Geometry check sheet. Reference: the model listing, model coordinates, mm. Face numbers are marked on the shaded views. Coordinates: 2 decimals unless noted, no trailing zeros. Write each loop counter-clockwise with the first axis right and the second up, starting at its lowest first coordinate (ties: lowest second). Pieces come first, ordered by that corner, then holes. Notation, with made-up numbers: (24, 2) -> (77, 2) arc R27 cw to (77, 41) -> close; hole circle Ø4 at (87, 89). An arc over 180 degrees is marked (long way). Answer as CSV lines item,"result".
```python
from build123d import *

# Parameters (mm, degrees)
EXTRUDE_1_DEPTH     = 3.6
SKETCH_2_W          = 40
SKETCH_2_H          = 20
CUT_EXTRUDE_1_DEPTH = 10


with BuildPart() as part:
    # 草图1 → 凸台-拉伸1 (new body)
    with BuildSketch(Plane.XY):
        Polygon((-95, 75.172935312), (-74.85, 75.172935312), (-74.85, 78.772935312), (-27.35, 78.772935312), (-27.35, 75.172935312), (20.15, 75.172935312), (20.15, 78.772935312), (67.65, 78.772935312), (67.65, 75.172935312), (87.799257887, 75), (87.799257887, 56.25), (91.399257887, 56.25), (91.399257887, 18.75), (87.799257887, 18.75), (87.799257887, -18.75), (91.399257887, -18.75), (91.399257887, -56.25), (87.799257887, -56.25), (87.799257887, -75), (67.65, -75), (67.65, -78.6), (20.15, -78.6), (20.15, -75), (-27.35, -75), (-27.35, -78.6), (-74.85, -78.6), (-74.85, -75), (-94.999257886, -74.827064673), (-95, -56.077064688), (-98.6, -56.077064688), (-98.6, -18.577064688), (-95, -18.577064688), (-95, 18.922935312), (-98.6, 18.922935312), (-98.6, 56.422935312), (-95, 56.422935312), align=None)
    extrude(amount=EXTRUDE_1_DEPTH)

    # 草图2 → 切除-拉伸1 (cut)
    with BuildSketch(Plane(origin=(0, 0, 0), x_dir=(-1, 0, 0), z_dir=(0, 0, -1))):
        Rectangle(SKETCH_2_W, SKETCH_2_H)
    extrude(amount=-CUT_EXTRUDE_1_DEPTH, mode=Mode.SUBTRACT)


solid = part.part
```
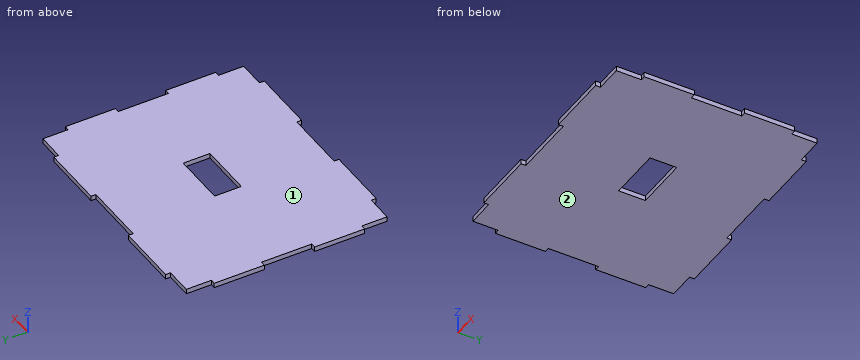
Item 1: Release check for a two-part mould opening along Z. For the marked faces 1 and 2 record: +Z half, -Z half, draft (parallel to the pull), parting line (faces both ways), or undercut.
Responses:
face 1,"+Z half"
face 2,"-Z half"
Item 2: Thickness scan on probe 1 along Y at (x, z) = (-17, 2.15); probe 2 along X at (y, z) = (9, 2.45); probe 3 along Y at (x, z) = (-26, 0.45). Record the ranges inside material, lowest first.
Responses:
probe 1,"y = -75 to -10, 10 to 75.17"
probe 2,"x = -95 to -20, 20 to 87.8"
probe 3,"y = -75 to 75.17"
Item 3: Cross-section at A-A, the plane y = -1.5. Record the cut outline in (x, z), plus the area to 3 significant figures.
Responses:
outline,"(-95, 0) -> (-20, 0) -> (-20, 3.6) -> (-95, 3.6) -> close; (20, 0) -> (87.8, 0) -> (87.8, 3.6) -> (20, 3.6) -> close"
area,"514 mm2"
Item 4: Cross-section at B-B, the plane x = 74. Record the cut outline in (y, z), plus the area to 3 significant figures.
Responses:
outline,"(-75, 0) -> (75.12, 0) -> (75.12, 3.6) -> (-75, 3.6) -> close"
area,"540 mm2"
Item 5: Depth check by flat-ended pin: pin 1 Ø1.8 at (y, z) = (-62.5, 2) entering from -X; pin 2 Ø1.1 at (x, z) = (88.5, 1.5) entering from +Y; pin 3 Ø2 at (y, z) = (-1.5, 3) entering from +X. Enter the tip coordinate at first touch or a pass-through.
Responses:
pin 1,"stops at x = -95"
pin 2,"stops at y = 56.25"
pin 3,"stops at x = 87.8"
Item 6: Cross-section at C-C, the plane x = -85. Record the cut outline in (y, z).
Responses:
outline,"(-74.91, 0) -> (75.17, 0) -> (75.17, 3.6) -> (-74.91, 3.6) -> close"
